from build123d import *

# Parameters (mm, degrees)
SKETCH_2_W           = 150
SKETCH_2_H           = 160
EXTRUDE_1_DEPTH      = 7
FILLET_1_R           = 5
SKETCH_3_R           = 1.65
CUT_EXTRUDE_1_DEPTH  = 8
SKETCH_6_R           = 2.02
SKETCH_6_R_2         = 2.2
CUT_EXTRUDE_2_DEPTH  = 8
SKETCH_9_R           = 3.15
CUT_EXTRUDE_4_DEPTH  = 3.5
SKETCH_10_R          = 3.75
CUT_EXTRUDE_5_DEPTH  = 4.2
CUT_EXTRUDE_6_DEPTH  = 8
SKETCH_12_R          = 1.65
CUT_EXTRUDE_7_DEPTH  = 50
SKETCH_14_R          = 3
CUT_EXTRUDE_9_DEPTH  = 3.3
SKETCH_15_R          = 1.65
CUT_EXTRUDE_10_DEPTH = 8
SKETCH_16_R          = 3
CUT_EXTRUDE_11_DEPTH = 3.3


with BuildPart() as part:
    # 草图2 → 凸台-拉伸1 (new body)
    with BuildSketch(Plane(origin=(0, 0, 0), x_dir=(1, 0, 0), z_dir=(0, 1, 0))):
        Rectangle(SKETCH_2_W, SKETCH_2_H)
    extrude(amount=EXTRUDE_1_DEPTH)

    # 圆角1
    fillet_1_edges = [part.edges().sort_by_distance(p)[0] for p in [
        (75, 3.5, 80),
        (-75, 3.5, 80),
        (-75, 3.5, -80),
        (75, 3.5, -80),
    ]]
    fillet(fillet_1_edges, radius=FILLET_1_R)

    # 草图3 → 切除-拉伸1 (cut, through all)
    with BuildSketch(Plane(origin=(0, 7, 0), x_dir=(1, 0, 0), z_dir=(0, 1, 0))):
        with Locations((-65, -35)):
            Circle(SKETCH_3_R)
        with Locations((-41, -35)):
            Circle(SKETCH_3_R)
        with Locations((-41, -65)):
            Circle(SKETCH_3_R)
        with Locations((-65, -65)):
            Circle(SKETCH_3_R)
        with Locations((65, -65)):
            Circle(SKETCH_3_R)
        with Locations((41, -65)):
            Circle(SKETCH_3_R)
        with Locations((41, -35)):
            Circle(SKETCH_3_R)
        with Locations((65, -35)):
            Circle(SKETCH_3_R)
        with Locations((-15, -40)):
            Circle(SKETCH_3_R)
        with Locations((-15, -60)):
            Circle(SKETCH_3_R)
        with Locations((15, -60)):
            Circle(SKETCH_3_R)
        with Locations((15, -40)):
            Circle(SKETCH_3_R)
    extrude(amount=-CUT_EXTRUDE_1_DEPTH, mode=Mode.SUBTRACT)

    # 草图6 → 切除-拉伸2 (cut, through all)
    with BuildSketch(Plane(origin=(0, 7, 0), x_dir=(1, 0, 0), z_dir=(0, 1, 0))):
        with Locations((12, 74)):
            Circle(SKETCH_6_R)
        with Locations((12, 56)):
            Circle(SKETCH_6_R_2)
        with Locations((-12, 56)):
            Circle(SKETCH_6_R_2)
        with Locations((-12, 74)):
            Circle(SKETCH_6_R)
    extrude(amount=-CUT_EXTRUDE_2_DEPTH, mode=Mode.SUBTRACT)

    # 草图9 → 切除-拉伸4 (cut)
    with BuildSketch(Plane.XZ):
        with Locations((-15, 60)):
            Circle(SKETCH_9_R)
        with Locations((-15, 40)):
            Circle(SKETCH_9_R)
        with Locations((15, 60)):
            Circle(SKETCH_9_R)
        with Locations((15, 40)):
            Circle(SKETCH_9_R)
        Polygon((-39.325684219, 67.9), (-37.651368439, 65), (-39.325684219, 62.1), (-42.674315781, 62.1), (-44.348631561, 65), (-42.674315781, 67.9), align=None)
        Polygon((61.651368439, 35), (63.325684219, 32.1), (66.674315781, 32.1), (68.348631561, 35), (66.674315781, 37.9), (63.325684219, 37.9), align=None)
        Polygon((37.651368439, 35), (39.325684219, 32.1), (42.674315781, 32.1), (44.348631561, 35), (42.674315781, 37.9), (39.325684219, 37.9), align=None)
        Polygon((61.651368439, 65), (63.325684219, 62.1), (66.674315781, 62.1), (68.348631561, 65), (66.674315781, 67.9), (63.325684219, 67.9), align=None)
        Polygon((37.651368439, 65), (39.325684219, 62.1), (42.674315781, 62.1), (44.348631561, 65), (42.674315781, 67.9), (39.325684219, 67.9), align=None)
        Polygon((-63.325684219, 67.9), (-61.651368439, 65), (-63.325684219, 62.1), (-66.674315781, 62.1), (-68.348631561, 65), (-66.674315781, 67.9), align=None)
        Polygon((-39.325684219, 37.9), (-37.651368439, 35), (-39.325684219, 32.1), (-42.674315781, 32.1), (-44.348631561, 35), (-42.674315781, 37.9), align=None)
        Polygon((-63.325684219, 37.9), (-61.651368439, 35), (-63.325684219, 32.1), (-66.674315781, 32.1), (-68.348631561, 35), (-66.674315781, 37.9), align=None)
    extrude(amount=-CUT_EXTRUDE_4_DEPTH, mode=Mode.SUBTRACT)

    # 草图10 → 切除-拉伸5 (cut)
    with BuildSketch(Plane.XZ):
        with Locations((12, -74)):
            Circle(SKETCH_10_R)
        with Locations((12, -56)):
            Circle(SKETCH_10_R)
        with Locations((-12, -56)):
            Circle(SKETCH_10_R)
        with Locations((-12, -74)):
            Circle(SKETCH_10_R)
    extrude(amount=-CUT_EXTRUDE_5_DEPTH, mode=Mode.SUBTRACT)

    # 草图11 → 切除-拉伸6 (cut, through all)
    with BuildSketch(Plane(origin=(0, 7, 0), x_dir=(1, 0, 0), z_dir=(0, 1, 0))):
        with BuildLine():
            Line((17, 27), (23, 27))
            ThreePointArc((23, 27), (25, 25), (23, 23))
            Line((23, 23), (17, 23))
            ThreePointArc((17, 23), (15, 25), (17, 27))
        make_face()
        with BuildLine():
            Line((-17, 27), (-23, 27))
            ThreePointArc((-23, 27), (-25, 25), (-23, 23))
            Line((-23, 23), (-17, 23))
            ThreePointArc((-17, 23), (-15, 25), (-17, 27))
        make_face()
        with BuildLine():
            Line((17, -27), (23, -27))
            ThreePointArc((23, -27), (25, -25), (23, -23))
            Line((23, -23), (17, -23))
            ThreePointArc((17, -23), (15, -25), (17, -27))
        make_face()
        with BuildLine():
            Line((-17, -27), (-23, -27))
            ThreePointArc((-23, -27), (-25, -25), (-23, -23))
            Line((-23, -23), (-17, -23))
            ThreePointArc((-17, -23), (-15, -25), (-17, -27))
        make_face()
    extrude(amount=-CUT_EXTRUDE_6_DEPTH, mode=Mode.SUBTRACT)

    # 草图12 → 切除-拉伸7 (cut)
    with BuildSketch(Plane.XZ):
        with Locations((-71, -65)):
            Circle(SKETCH_12_R)
        with Locations((-71, 15)):
            Circle(SKETCH_12_R)
        with Locations((71, 15)):
            Circle(SKETCH_12_R)
        with Locations((71, -65)):
            Circle(SKETCH_12_R)
    extrude(amount=-CUT_EXTRUDE_7_DEPTH, mode=Mode.SUBTRACT)

    # 草图14 → 切除-拉伸9 (cut)
    with BuildSketch(Plane.XZ):
        with Locations((-71, -65)):
            Circle(SKETCH_14_R)
        with Locations((-71, 15)):
            Circle(SKETCH_14_R)
        with Locations((71, -65)):
            Circle(SKETCH_14_R)
        with Locations((71, 15)):
            Circle(SKETCH_14_R)
    extrude(amount=-CUT_EXTRUDE_9_DEPTH, mode=Mode.SUBTRACT)

    # 草图15 → 切除-拉伸10 (cut, through all)
    with BuildSketch(Plane.XZ):
        with Locations((0, 76)):
            Circle(SKETCH_15_R)
    extrude(amount=-CUT_EXTRUDE_10_DEPTH, mode=Mode.SUBTRACT)

    # 草图16 → 切除-拉伸11 (cut)
    with BuildSketch(Plane.XZ):
        with Locations((0, 76)):
            Circle(SKETCH_16_R)
    extrude(amount=-CUT_EXTRUDE_11_DEPTH, mode=Mode.SUBTRACT)


solid = part.part
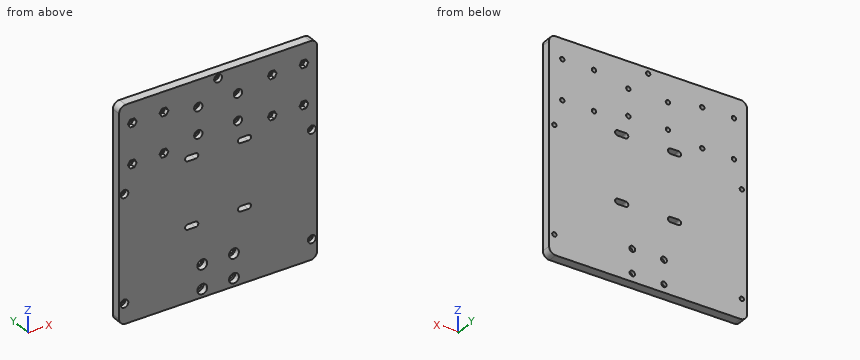
Geometry: final body of the model. Coordinates: model frame, mm. Coordinates: 2 decimals unless noted, no trailing zeros. Put each result on its own line as item: value. Start each with the question number.
Q1. Line query: line 1 (X direction, y = 5.1, z = 65); line 2 (Z direction, x = 64, y = 2); line 3 (X direction, y = 6, z = -56). Output: solid intervals per line, ascending.
Q2. Cut plane A-A, the plane y = 5.5. Give the number of separate pieces and of enclosed holes in the cut face, and give its area (3 significant figures).
Q3. Pin query (flat end, axial travel): pin 1 Ø5 at (x, z) = (12, -56) entering from -Y; pin 2 Ø5.5 at (x, z) = (-65, 35) entering from -Y; pin 3 Ø8 at (x, z) = (0, 76) entering from -Y; pin 4 Ø4 at (x, z) = (71, -65) entering from -Y. Return the tip coordinate at first contact, or that it passes through.
Filled sheet:
1. line 1: -75 to -66.65, -63.35 to -42.65, -39.35 to 39.35, 42.65 to 63.35, 66.65 to 75
1. line 2: -80 to 32.1, 37.9 to 62.1, 67.9 to 80
1. line 3: -75 to -14.2, -9.8 to 9.8, 14.2 to 75
2. separate pieces: 1
2. enclosed holes: 25
2. area: 23,600 mm²
3. pin 1: y = 4.2
3. pin 2: y = 3.5
3. pin 3: y = 0
3. pin 4: y = 3.3
